from build123d import *

# Parameters (mm, degrees)
F0_W     = 150
F0_H     = 38
F0_R     = 6
F0_R_2   = 8.25
F1_DEPTH = 5
F2_R     = 5


with BuildPart() as f1:
    # F0 (on Front) → F1 (new body)
    with BuildSketch(Plane.XZ):
        Rectangle(F0_W, F0_H)
        with Locations((-60, 0)):
            Circle(F0_R, mode=Mode.SUBTRACT)
        with Locations((-40, 0)):
            Circle(F0_R, mode=Mode.SUBTRACT)
        Circle(F0_R_2, mode=Mode.SUBTRACT)
        with Locations((30, 0)):
            Circle(F0_R_2, mode=Mode.SUBTRACT)
        with Locations((60, 0)):
            Circle(F0_R_2, mode=Mode.SUBTRACT)
    extrude(amount=F1_DEPTH)

    # F2
    f2_edges = [f1.edges().sort_by_distance(p)[0] for p in [
        (-75, -2.5, 19),
        (-75, -2.5, -19),
        (75, -2.5, 19),
        (75, -2.5, -19),
    ]]
    fillet(f2_edges, radius=F2_R)


solid = f1.part
Source: CAD feature listing. Evaluate the final solid. Frame: model axes, mm. Round coordinates to 2 decimals unless told otherwise and drop trailing zeros. Write each loop counter-clockwise with the first axis right and the second up, starting at its lowest first coordinate (ties: lowest second). Pieces come first, ordered by that corner, then holes. Notation, with made-up numbers: M 81,18 L 110,18 A14 cw 110,27 Z; hole C 1.5,-22.75 d5. An arc over 180 degrees is marked long. One line per item, written item: value. Start each with the question number.
Item 1: Section query C-C (z = -4.5). Return the cut outline in (x, y).
Item 2: Section query A-A (x = 30). Return the cut outline in (y, z), plus the area to 4 significant figures.
Item 3: Mould query, pull axis Z, two halves, no side actions, for faces 1 (the cylindrical face through (-46, -2, 0)), 2 (the flat face through (75, -2, 0)), 3 (the cylindrical face through (7.62, -2.46, -3.16)), 4 (the cylindrical face through (73, -3, -18)). Classes: pulls with the +Z half, pulls with the -Z half, needs draft (parallel to the pull), parting line crosses it, or undercut.
Item 4: Ray query, L1, parallel to Z at x = 0, y = -1.25; L2, parallel to Z at x = -40, y = -1; L3, parallel to X at y = -4.1, z = 7.5. Return the intervals inside material, ascending. Write a range as from..to.
Item 5: Section query B-B (y = -2.8). Return the cut outline in (x, z).
Item 6: Section query D-D (x = -40). Return the cut outline in (y, z), plus the area to 3 significant figures.
Result set:
1. outline: M -75,-5 L -63.97,-5 L -63.97,0 L -75,0 Z; M -56.03,-5 L -43.97,-5 L -43.97,0 L -56.03,0 Z; M -36.03,-5 L -6.91,-5 L -6.91,0 L -36.03,0 Z; M 6.91,-5 L 23.09,-5 L 23.09,0 L 6.91,0 Z; M 36.91,-5 L 53.09,-5 L 53.09,0 L 36.91,0 Z; M 66.91,-5 L 75,-5 L 75,0 L 66.91,0 Z
2. outline: M -5,-19 L 0,-19 L 0,-8.25 L -5,-8.25 Z; M -5,8.25 L 0,8.25 L 0,19 L -5,19 Z
2. area: 107.5 mm²
3. face 1: undercut
3. face 2: needs draft
3. face 3: undercut
3. face 4: pulls with the -Z half
4. L1: z = -19..-8.25, 8.25..19
4. L2: z = -19..-6, 6..19
4. L3: x = -75..-3.44, 3.44..26.56, 33.44..56.56, 63.44..75
5. outline: M -75,-14 A5 ccw -70,-19 L 70,-19 A5 ccw 75,-14 L 75,14 A5 ccw 70,19 L -70,19 A5 ccw -75,14 Z; hole C -60,0 d12; hole C -40,0 d12; hole C 0,0 d16.5; hole C 30,0 d16.5; hole C 60,0 d16.5
6. outline: M -5,-19 L 0,-19 L 0,-6 L -5,-6 Z; M -5,6 L 0,6 L 0,19 L -5,19 Z
6. area: 130 mm²
